```python
from build123d import *

# Parameters (mm, degrees)
SKETCH1_W           = 21
SKETCH1_H           = 100
SKETCH1_R           = 1.75
BOSS_EXTRUDE1_DEPTH = 5
SKETCH2_W           = 100
SKETCH2_H           = 38
BOSS_EXTRUDE2_DEPTH = 14
SKETCH3_W           = 50
SKETCH3_H           = 5
BOSS_EXTRUDE3_DEPTH = 15
SKETCH4_R           = 1.75
CUT_EXTRUDE1_DEPTH  = 16
BOSS_EXTRUDE6_DEPTH = 15
SKETCH9_R           = 3.25
CUT_EXTRUDE3_DEPTH  = 36
SKETCH10_R          = 5.25
CUT_EXTRUDE4_DEPTH  = 9
CUT_EXTRUDE5_REACH  = 28.5
SKETCH11_W          = 5
SKETCH11_H          = 9.2
SKETCH12_R          = 1.75
CUT_EXTRUDE6_DEPTH  = 4
SKETCH13_W          = 100
SKETCH13_H          = 13
BOSS_EXTRUDE7_DEPTH = 30
SKETCH14_R          = 2.5
CUT_EXTRUDE7_DEPTH  = 39
CUT_EXTRUDE8_DEPTH  = 5
SKETCH16_R          = 2.1
CUT_EXTRUDE9_DEPTH  = 4
CHAMFER1_SIZE       = 1.6
CUT_EXTRUDE10_DEPTH = 39
CHAMFER2_SIZE       = 1.6
CHAMFER3_SIZE       = 5
SKETCH18_R          = 1.75
CUT_EXTRUDE11_DEPTH = 4
FILLET1_R           = 5
FILLET2_R           = 4
SKETCH19_W          = 13.3
SKETCH19_H          = 6.3
CUT_EXTRUDE12_DEPTH = 10.5
SKETCH20_R          = 1
CUT_EXTRUDE13_DEPTH = 3
CHAMFER4_SIZE       = 3
FILLET3_R           = 2
SKETCH22_W          = 13.3
SKETCH22_H          = 10.5
CUT_EXTRUDE14_DEPTH = 6.3
SKETCH23_R          = 1
CUT_EXTRUDE15_DEPTH = 3
CHAMFER5_SIZE       = 3


with BuildPart() as part:
    # Sketch1 → Boss-Extrude1 (new body)
    with BuildSketch(Plane(origin=(0, 0, 0), x_dir=(1, 0, 0), z_dir=(0, 1, 0))):
        Rectangle(SKETCH1_W, SKETCH1_H)
        with Locations((-7.5, 36)):
            Circle(SKETCH1_R, mode=Mode.SUBTRACT)
        with Locations((7.5, 36)):
            Circle(SKETCH1_R, mode=Mode.SUBTRACT)
        with Locations((-7.5, 20)):
            Circle(SKETCH1_R, mode=Mode.SUBTRACT)
        with Locations((7.5, 20)):
            Circle(SKETCH1_R, mode=Mode.SUBTRACT)
        with Locations((7.5, -20)):
            Circle(SKETCH1_R, mode=Mode.SUBTRACT)
        with Locations((-7.5, -20)):
            Circle(SKETCH1_R, mode=Mode.SUBTRACT)
        with Locations((7.5, -36)):
            Circle(SKETCH1_R, mode=Mode.SUBTRACT)
        with Locations((-7.5, -36)):
            Circle(SKETCH1_R, mode=Mode.SUBTRACT)
    extrude(amount=BOSS_EXTRUDE1_DEPTH)

    # Sketch2 → Boss-Extrude2 (add)
    with BuildSketch(Plane(origin=(10.5, 0, 0), x_dir=(0, 0, -1), z_dir=(1, 0, 0))):
        with Locations((0, -14)):
            Rectangle(SKETCH2_W, SKETCH2_H)
    extrude(amount=BOSS_EXTRUDE2_DEPTH)

    # Sketch3 → Boss-Extrude3 (add)
    with BuildSketch(Plane(origin=(24.5, 0, 0), x_dir=(0, 0, -1), z_dir=(1, 0, 0))):
        with Locations((0, -20.5)):
            Rectangle(SKETCH3_W, SKETCH3_H)
    extrude(amount=BOSS_EXTRUDE3_DEPTH)

    # Sketch4 → Cut-Extrude1 (cut, through all)
    with BuildSketch(Plane(origin=(0, -18, 0), x_dir=(1, 0, 0), z_dir=(0, 1, 0))):
        with Locations((34.5, 15)):
            Circle(SKETCH4_R)
        with Locations((34.5, -15)):
            Circle(SKETCH4_R)
    extrude(amount=-CUT_EXTRUDE1_DEPTH, mode=Mode.SUBTRACT)

    # Sketch8 → Boss-Extrude6 (add)
    with BuildSketch(Plane(origin=(24.5, 0, 0), x_dir=(0, 0, -1), z_dir=(1, 0, 0))):
        Polygon((-50, -6.5), (-25, -6.5), (-25, -33), (-50, -33), (-50, -30), (-29.5, -30), (-29.5, -9.5), (-50, -9.5), align=None)
        Polygon((29.5, -30), (29.5, -9.5), (50, -9.5), (50, -6.5), (25, -6.5), (25, -33), (50, -33), (50, -30), align=None)
    extrude(amount=BOSS_EXTRUDE6_DEPTH)

    # Sketch9 → Cut-Extrude3 (cut, through all)
    with BuildSketch(Plane(origin=(24.5, 0, 0), x_dir=(0, 0, -1), z_dir=(1, 0, 0))):
        with Locations((-39.75, -19.75)):
            Circle(SKETCH9_R)
        with Locations((39.75, -19.75)):
            Circle(SKETCH9_R)
    extrude(amount=-CUT_EXTRUDE3_DEPTH, mode=Mode.SUBTRACT)

    # Sketch10 → Cut-Extrude4 (cut)
    with BuildSketch(Plane.ZY.offset(-10.5)):
        with Locations((-39.75, -19.75)):
            Circle(SKETCH10_R)
        with Locations((39.75, -19.75)):
            Circle(SKETCH10_R)
    extrude(amount=-CUT_EXTRUDE4_DEPTH, mode=Mode.SUBTRACT)

    # Sketch11 → Cut-Extrude5 (cut, up to next)
    with BuildSketch(Plane(origin=(0, -6.5, 0), x_dir=(1, 0, 0), z_dir=(0, 1, 0)), mode=Mode.PRIVATE) as cut_extrude5_sk1:
        with Locations((37, -39.75)):
            Rectangle(SKETCH11_W, SKETCH11_H)
    cut_extrude5_tool1 = extrude(cut_extrude5_sk1.sketch, amount=-CUT_EXTRUDE5_REACH, mode=Mode.PRIVATE) & part.part
    add(cut_extrude5_tool1.solids().sort_by_distance((37, -6.5, 39.75))[0], mode=Mode.SUBTRACT)
    # Sketch11 → Cut-Extrude5 (cut, up to next)
    with BuildSketch(Plane(origin=(0, -6.5, 0), x_dir=(1, 0, 0), z_dir=(0, 1, 0)), mode=Mode.PRIVATE) as cut_extrude5_sk2:
        with Locations((37, 39.75)):
            Rectangle(SKETCH11_W, SKETCH11_H)
    cut_extrude5_tool2 = extrude(cut_extrude5_sk2.sketch, amount=-CUT_EXTRUDE5_REACH, mode=Mode.PRIVATE) & part.part
    add(cut_extrude5_tool2.solids().sort_by_distance((37, -6.5, -39.75))[0], mode=Mode.SUBTRACT)

    # Sketch12 → Cut-Extrude6 (cut, through all)
    with BuildSketch(Plane(origin=(0, -30, 0), x_dir=(1, 0, 0), z_dir=(0, 1, 0))):
        with Locations((32, -39.75)):
            Circle(SKETCH12_R)
        with Locations((32, 39.75)):
            Circle(SKETCH12_R)
    extrude(amount=-CUT_EXTRUDE6_DEPTH, mode=Mode.SUBTRACT)

    # Sketch13 → Boss-Extrude7 (add)
    with BuildSketch(Plane.ZY.offset(10.5)):
        with Locations((0, -1.5)):
            Rectangle(SKETCH13_W, SKETCH13_H)
    extrude(amount=BOSS_EXTRUDE7_DEPTH)

    # Sketch14 → Cut-Extrude7 (cut, through all)
    with BuildSketch(Plane(origin=(0, 5, 0), x_dir=(1, 0, 0), z_dir=(0, 1, 0))):
        with Locations((-17.4375, 41.8075)):
            Circle(SKETCH14_R)
        with Locations((-31.15, -42.205)):
            Circle(SKETCH14_R)
    extrude(amount=-CUT_EXTRUDE7_DEPTH, mode=Mode.SUBTRACT)

    # Sketch15 → Cut-Extrude8 (cut)
    with BuildSketch(Plane.XZ.offset(8)):
        Polygon((-27.05, 44.572136104), (-31.15, 46.939272207), (-35.25, 44.572136104), (-35.25, 39.837863896), (-31.15, 37.470727793), (-27.05, 39.837863896), align=None)
        Polygon((-13.3375, -44.174636104), (-13.3375, -39.440363896), (-17.4375, -37.073227793), (-21.5375, -39.440363896), (-21.5375, -44.174636104), (-17.4375, -46.541772207), align=None)
    extrude(amount=-CUT_EXTRUDE8_DEPTH, mode=Mode.SUBTRACT)

    # Sketch16 → Cut-Extrude9 (cut)
    with BuildSketch(Plane(origin=(0, 5, 0), x_dir=(1, 0, 0), z_dir=(0, 1, 0))):
        with Locations((19.5, 39.75)):
            Circle(SKETCH16_R)
        with Locations((19.5, -39.75)):
            Circle(SKETCH16_R)
    extrude(amount=-CUT_EXTRUDE9_DEPTH, mode=Mode.SUBTRACT)

    # Chamfer1
    chamfer1_edges = [part.edges().sort_by_distance(p)[0] for p in [
        (-9.25, 5, -36),
        (5.75, 5, -36),
        (-9.25, 5, -20),
        (5.75, 5, -20),
        (5.75, 5, 20),
        (-9.25, 5, 20),
        (5.75, 5, 36),
        (-9.25, 5, 36),
    ]]
    chamfer(chamfer1_edges, length=CHAMFER1_SIZE)

    # Sketch17 → Cut-Extrude10 (cut, through all)
    with BuildSketch(Plane(origin=(0, 5, 0), x_dir=(1, 0, 0), z_dir=(0, 1, 0))):
        Polygon((-40.5, 20), (-15.5, 7.5), (-15.5, -7.5), (-40.5, -20), align=None)
    extrude(amount=-CUT_EXTRUDE10_DEPTH, mode=Mode.SUBTRACT)

    # Chamfer2
    chamfer2_edges = [part.edges().sort_by_distance(p)[0] for p in [
        (30.25, -33, 39.75),
        (30.25, -33, -39.75),
    ]]
    chamfer(chamfer2_edges, length=CHAMFER2_SIZE)

    # Chamfer3
    chamfer3_edges = [part.edges().sort_by_distance(p)[0] for p in [
        (10.5, -33, 0),
    ]]
    chamfer(chamfer3_edges, length=CHAMFER3_SIZE)

    # Sketch18 → Cut-Extrude11 (cut)
    with BuildSketch(Plane(origin=(0, 1, 0), x_dir=(1, 0, 0), z_dir=(0, 1, 0))):
        with Locations((19.5, 39.75)):
            Circle(SKETCH18_R)
        with Locations((19.5, -39.75)):
            Circle(SKETCH18_R)
    extrude(amount=-CUT_EXTRUDE11_DEPTH, mode=Mode.SUBTRACT)

    # Fillet1
    fillet1_edges = [part.edges().sort_by_distance(p)[0] for p in [
        (-40.5, -1.5, -50),
        (-40.5, -1.5, 50),
        (-40.5, -1.5, 20),
        (-40.5, -1.5, -20),
        (-15.5, -1.5, -7.5),
        (-15.5, -1.5, 7.5),
    ]]
    fillet(fillet1_edges, radius=FILLET1_R)

    # Fillet2
    fillet2_edges = [part.edges().sort_by_distance(p)[0] for p in [
        (32, -6.5, -25),
        (32, -33, -25),
        (32, -33, 25),
        (32, -6.5, 25),
    ]]
    fillet(fillet2_edges, radius=FILLET2_R)

    # Sketch19 → Cut-Extrude12 (cut)
    with BuildSketch(Plane(origin=(24.5, 0, 0), x_dir=(0, 0, -1), z_dir=(1, 0, 0))):
        with Locations((0, 1.85)):
            Rectangle(SKETCH19_W, SKETCH19_H)
    extrude(amount=-CUT_EXTRUDE12_DEPTH, mode=Mode.SUBTRACT)

    # Sketch20 → Cut-Extrude13 (cut)
    with BuildSketch(Plane(origin=(0, -1.3, 0), x_dir=(1, 0, 0), z_dir=(0, 1, 0))):
        with Locations((18.5, 3.25)):
            Circle(SKETCH20_R)
        with Locations((18.5, -3.25)):
            Circle(SKETCH20_R)
    extrude(amount=-CUT_EXTRUDE13_DEPTH, mode=Mode.SUBTRACT)

    # Chamfer4
    chamfer4_edges = [part.edges().sort_by_distance(p)[0] for p in [
        (14, 5, 0),
    ]]
    chamfer(chamfer4_edges, length=CHAMFER4_SIZE)

    # Fillet3
    fillet3_edges = [part.edges().sort_by_distance(p)[0] for p in [
        (24.5, 5, 28.325),
        (24.5, 5, -28.325),
    ]]
    fillet(fillet3_edges, radius=FILLET3_R)

    # Sketch22 → Cut-Extrude14 (cut)
    with BuildSketch(Plane(origin=(0, 5, 0), x_dir=(1, 0, 0), z_dir=(0, 1, 0))):
        with Locations((-20.15, -44.75)):
            Rectangle(SKETCH22_W, SKETCH22_H)
    extrude(amount=-CUT_EXTRUDE14_DEPTH, mode=Mode.SUBTRACT)

    # Sketch23 → Cut-Extrude15 (cut)
    with BuildSketch(Plane(origin=(0, -1.3, 0), x_dir=(1, 0, 0), z_dir=(0, 1, 0))):
        with Locations((-23.4, -44)):
            Circle(SKETCH23_R)
        with Locations((-16.9, -44)):
            Circle(SKETCH23_R)
    extrude(amount=-CUT_EXTRUDE15_DEPTH, mode=Mode.SUBTRACT)

    # Chamfer5
    chamfer5_edges = [part.edges().sort_by_distance(p)[0] for p in [
        (-20.15, 5, 39.5),
    ]]
    chamfer(chamfer5_edges, length=CHAMFER5_SIZE)


solid = part.part
```
Part model, mm, in its own coordinate system. A direction names the side the tool comes from. Round coordinates to 2 decimals unless told otherwise and drop trailing zeros. Write each loop counter-clockwise with the first axis right and the second up, starting at its lowest first coordinate (ties: lowest second). Pieces come first, ordered by that corner, then holes.
Item 1: Cut at A-A, the plane z = 15. Give the cut face in (x, y), plus the area to 3 significant figures.
Results:
outline: (-30.5, -8) - (-10.5, -8) - (-10.5, 0) - (10.5, 0) - (10.5, -28) - (15.5, -33) - (24.5, -33) - (24.5, -23) - (32.75, -23) - (32.75, -18) - (24.5, -18) - (24.5, 3) arc R2 ccw to (22.5, 5) - (-30.5, 5) - close; (36.25, -23) - (39.5, -23) - (39.5, -18) - (36.25, -18) - close
area: 941 mm2
Item 2: Two-plate mould, pull along X, no slides. Class faces 5 (the flat face through (39.5, -22, 3)), 6 (the cylindrical face through (-7.728, 1.676, -21.735)), 7 (the flat face through (30, -30, 40)): +X half, -X half, draft (parallel to the pull), parting line (faces both ways), or undercut.
Results:
face 5: +X half
face 6: undercut
face 7: draft
Item 3: Drop flat-ended pins along their axis: pin 1 Ø0.6 at (x, z) = (18.5, -3.5) entering from +Y; pin 2 Ø1.5 at (y, z) = (-2.5, -19.5) entering from -X (3 decimals); pin 3 Ø8 at (y, z) = (-28.5, -2.5) entering from +X; pin 4 Ø5 at (y, z) = (-19.75, 39.75) entering from +X. Give the stop position or say it passes through.
Results:
pin 1: stops at y = -4.3
pin 2: stops at x = -39.615
pin 3: stops at x = 24.5
pin 4: passes through
Item 4: Cut at B-B, the plane x = 7.5. Give the cut face in (y, z).
Results:
outline: (0, -50) - (5, -50) - (5, -39.35) - (3.4, -37.75) - (0, -37.75) - close; (0, -34.25) - (3.4, -34.25) - (5, -32.65) - (5, -23.35) - (3.4, -21.75) - (0, -21.75) - close; (0, -18.25) - (3.4, -18.25) - (5, -16.65) - (5, 16.65) - (3.4, 18.25) - (0, 18.25) - close; (0, 21.75) - (3.4, 21.75) - (5, 23.35) - (5, 32.65) - (3.4, 34.25) - (0, 34.25) - close; (0, 37.75) - (3.4, 37.75) - (5, 39.35) - (5, 50) - (0, 50) - close
Item 5: Probe L1, parallel to Z at x = 18.5, y = -3.4; L2, parallel to Z at x = 19, y = -19.5; L3, parallel to Z at x = 19.5, y = -0.7. List the from-to ranges inside material, lowest first.
Results:
L1: z = -50 to -4.25, -2.25 to 2.25, 4.25 to 50
L2: z = -50 to -44.99, -34.51 to 34.51, 44.99 to 50
L3: z = -50 to -41.5, -38 to -6.65, 6.65 to 38, 41.5 to 50
Item 6: Cut at C-C, the plane y = -21.5. Give the cut face in (x, z), plus the area to 3 significant figures.
Results:
outline: (10.5, -50) - (24.5, -50) - (24.5, -42.49) - (19.5, -42.49) - (19.5, -44.7) - (10.5, -44.7) - close; (10.5, -34.8) - (19.5, -34.8) - (19.5, -37.01) - (24.5, -37.01) - (24.5, -29.5) - (39.5, -29.5) - (39.5, 29.5) - (24.5, 29.5) - (24.5, 37.01) - (19.5, 37.01) - (19.5, 34.8) - (10.5, 34.8) - close; (10.5, 44.7) - (19.5, 44.7) - (19.5, 42.49) - (24.5, 42.49) - (24.5, 50) - (10.5, 50) - close; hole circle Ø3.5 at (34.5, -15); hole circle Ø3.5 at (34.5, 15)
area: 2,030 mm2
Item 7: Cut at D-D, the plane z = -20. Give the cut face in (x, y).
Results:
outline: (-39.43, -8) - (-10.5, -8) - (-10.5, 0) - (-9.25, 0) - (-9.25, 3.4) - (-10.85, 5) - (-39.43, 5) - close; (-5.75, 0) - (5.75, 0) - (5.75, 3.4) - (4.15, 5) - (-4.15, 5) - (-5.75, 3.4) - close; (9.25, 0) - (10.5, 0) - (10.5, -28) - (15.5, -33) - (24.5, -33) - (24.5, -23) - (39.5, -23) - (39.5, -18) - (24.5, -18) - (24.5, 3) arc R2 ccw to (22.5, 5) - (10.85, 5) - (9.25, 3.4) - close
Item 8: Which spindle directions (+Z, -Z, +X, -X, +Y, -Y) get a long thin tool onto all of the face, cutting with end or side? Do faces 1 (the flat face through (-15, -8, -1)), 2 (the flat face through (30, -6.5, 40)), 3 (the flat face through (37, -8, -44.35)), 4 (the cylindrical face through (30.6, -30.7, 40.8)). Say none if no direction does.
Results:
face 1: +Z, -Z, -X, -Y
face 2: +Z, -Z, +X, +Y
face 3: +X, +Y
face 4: -Y
